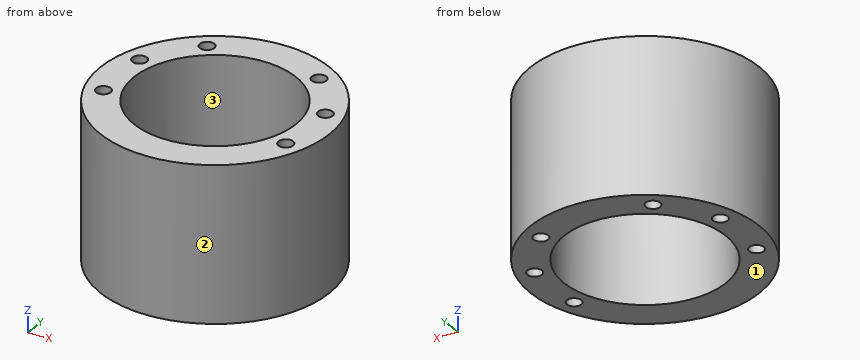
from build123d import *

# Parameters (mm, degrees)
SKETCH1_R           = 49.53
SKETCH1_R_2         = 35
SKETCH1_R_3         = 3.175
BOSS_EXTRUDE1_DEPTH = 67


with BuildPart() as part:
    # Sketch1 → Boss-Extrude1 (new body)
    with BuildSketch(Plane.XY):
        Circle(SKETCH1_R)
        Circle(SKETCH1_R_2, mode=Mode.SUBTRACT)
        with Locations((40.104626484, 12.474731845)):
            Circle(SKETCH1_R_3, mode=Mode.SUBTRACT)
        with Locations((-39.397117561, -14.555656215)):
            Circle(SKETCH1_R_3, mode=Mode.SUBTRACT)
        with Locations((39.397117561, -14.555656215)):
            Circle(SKETCH1_R_3, mode=Mode.SUBTRACT)
        with Locations((-24.189576015, 34.334594977)):
            Circle(SKETCH1_R_3, mode=Mode.SUBTRACT)
        with Locations((-40.104626484, 12.474731845)):
            Circle(SKETCH1_R_3, mode=Mode.SUBTRACT)
        with Locations((24.189576015, 34.334594977)):
            Circle(SKETCH1_R_3, mode=Mode.SUBTRACT)
    extrude(amount=-BOSS_EXTRUDE1_DEPTH)


solid = part.part
Could you check a few things on this model? Use its own coordinates, in mm. Face numbers are marked on the shaded views. Round coordinates to 2 decimals unless told otherwise and drop trailing zeros. Order: outer loops, then holes, each group sorted by start corner. A loop starts at its lowest first (then second) coordinate and runs counter-clockwise, first axis right, second up.
Q1. Imagine slicing it at C-C, the plane z = -60. List the corners of the cut face in (x, y) for me (3 decimals), then the cut area to 3 significant figures.
Geometry says:
outline: circle Ø99.06 at (0, 0); hole circle Ø6.35 at (-40.105, 12.475); hole circle Ø6.35 at (-39.397, -14.556); hole circle Ø70 at (0, 0); hole circle Ø6.35 at (-24.19, 34.335); hole circle Ø6.35 at (24.19, 34.335); hole circle Ø6.35 at (39.397, -14.556); hole circle Ø6.35 at (40.105, 12.475)
area: 3,670 mm2
Q2. Thinking about a two-plate mould opening in Y: for the marked faces 1, 2 and 3, which applies, released by +Y, released by -Y, zero draft, split by the parting line, or undercut?
Geometry says:
face 1: zero draft
face 2: split by the parting line
face 3: undercut
Q3. I'm going to push flat-ended pins straight in: P1, Ø10, axis at y = -22, z = -30, coming from the -X side; P2, Ø4, axis at x = 21, z = -24.5, coming from the +Y side; P3, Ø3, axis at y = 22.5, z = -59.5, coming from the -X side. Where does each tip first touch, or does it pass through?
Geometry says:
P1: stops at x = -46.52
P2: stops at y = 45.74
P3: stops at x = -44.86
Q4. Please list where these lines run through material, in increasing order: probe 1 along Y at (x, z) = (-24, -21); probe 2 along Y at (x, z) = (39.5, -56.5); probe 3 along Y at (x, z) = (0, -45).
Geometry says:
probe 1: y = -43.33 to -25.48, 25.48 to 31.17, 37.5 to 43.33
probe 2: y = -29.88 to -17.73, -11.38 to 9.36, 15.59 to 29.88
probe 3: y = -49.53 to -35, 35 to 49.53
Q5. Imagine slicing it at A-A, the plane x = 0. List the corners of the cut face in (y, z) for me.
Geometry says:
outline: (-49.53, -67) - (-35, -67) - (-35, 0) - (-49.53, 0) - close; (35, -67) - (49.53, -67) - (49.53, 0) - (35, 0) - close
